Autodesk Inventor part; units mm, degrees
ref_plane "YZ Plane" through (0, 0, 0) normal (1, 0, 0) x (0, 1, 0)
ref_plane "XZ Plane" through (0, 0, 0) normal (0, 1, 0) x (-1, 0, 0)
ref_plane "XY Plane" through (0, 0, 0) normal (0, 0, 1) x (1, 0, 0)
ref_plane "Work Plane1" through (0, 0, 0) normal (0, 0, 1) x (1, 0, 0)
sketch "Sketch1" plane through (0, 0, 0) normal (0, 0, 1) x (1, 0, 0)
  circle A0 centre (0, 0) radius 7.5
  line L0 (-30, 28) -> (-28, 30)
  line L1 (-30, -28) -> (-30, 28)
  line L2 (-28, -30) -> (-30, -28)
  line L3 (28, -30) -> (-28, -30)
  line L4 (30, -28) -> (28, -30)
  line L5 (30, 28) -> (30, -28)
  line L6 (28, 30) -> (30, 28)
  line L7 (-28, 30) -> (28, 30)
  circle A1 centre (-25, 0) radius 1.3
  circle A2 centre (25, 0) radius 1.3
extrude "Extrusion1" add sketch "Sketch1" along normal blind 12 contours A0 | L0 L7 L6 L5 L4 L3 L2 L1 | A1 | A2
sketch "Sketch2" plane through (0, 0, 12) normal (0, 0, 1) x (1, 0, 0)
  point P0 (0, 0)
sketch "Sketch3" plane through (30, -28, 0) normal (1, 0, 0) x (0, 0, -1)
  line L0 (0, 56) -> (0, 0)
  line L1 (0, 56) -> (-12, 56)
  line L2 (-12, 0) -> (-12, 56)
  line L3 (0, 0) -> (-12, 0)
  line L4 (-12, 0) -> (-12, 56)
  line L5 (0, 47.2331) -> (-12, 47.2331)
  line L6 (-12, 47.2331) -> (-12, 36.3051)
  line L7 (-12, 36.3051) -> (0, 36.3051)
  line L8 (0, 36.3051) -> (0, 47.2331)
  line L9 (0, 56) -> (0, 0)
  line L10 (0, 10.2066) -> (-12, 10.2066)
  line L11 (-12, 10.2066) -> (-12, 18.9489)
  line L12 (-12, 18.9489) -> (0, 18.9489)
  line L13 (0, 18.9489) -> (0, 10.2066)
  point P0 (0, 28)
extrude "Extrusion2" add sketch "Sketch3" along normal blind 14 contours L0 L7 L2 L5 | L0 L10 L2 L12
sketch "Sketch4" plane through (30, 19.2331, 12) normal (0, 1, 0) x (1, 0, 0)
  line L0 (0, 0) -> (0, 12)
  line L1 (0, 0) -> (14, 0)
  line L2 (14, 12) -> (14, 0)
  line L3 (0, 12) -> (14, 12)
  circle A0 centre (7, 5) radius 1.5
  point P0 (-30, 12)
  dimension "d4" = 3
extrude "Extrusion3" cut sketch "Sketch4" against normal through all contours A0
pattern_circular "Circular Pattern1" count 2 over 90 about axis through (0, 0, 0) along (0, 0, 1) of "Extrusion2", "Extrusion3"
properties part number "00_XY_stage-CHUO_SEIKI_LD-647-R1-Middle"
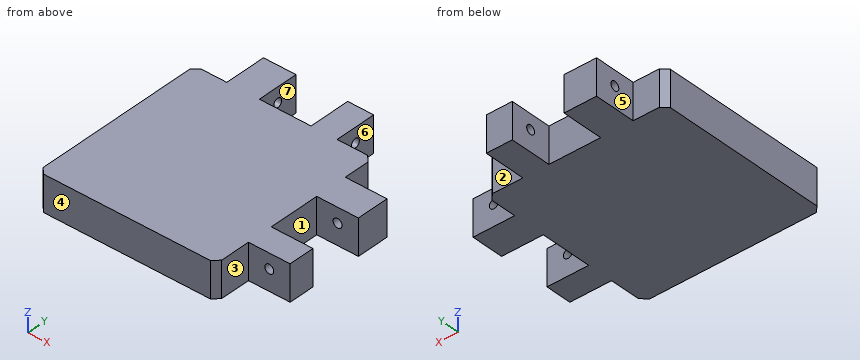
The model under review builds one solid part; all positions refer to its coordinate system, in mm. Face numbers are marked on the shaded views. A direction names the side the tool comes from. Round coordinates to 2 decimals unless told otherwise and drop trailing zeros. Loops run counter-clockwise (first coordinate to the right, second up) from the corner with the lowest first, then second, coordinate; pieces in that order, holes last. Notation, with made-up numbers: (-21, 3) - (-11, 3) arc R33 cw to (-11, 37) - close; hole circle Ø2 at (-29.75, 71.5). An arc over 180 degrees is marked (long way). Write each question's results on one line, items separated by ' | '. Start each with the question number.
Q1. Tool access review of the marked faces 5, 6 and 7: name each direction out of +Z, -Z, +X, -X, +Y, -Y from which nothing blocks a thin tool from reaching the whole face with its end or side.
Q2. Draft analysis for pull direction Y (two halves, no side actions). For the marked faces 1, 2, 3 and 4, state which applies: pulls with the +Y half, pulls with the -Y half, needs draft (parallel to the pull), parting line crosses it, or undercut.
Q3. Take a section at C-C on z = 4. Give the boundary of the cut face in (x, y).
Q4. Take a section at D-D on x = -23.5. Give the boundary of the cut face in (y, z), plus the area to 3 significant figures.
Q5. Take a section at B-B on y = 37. Give the boundary of the cut face in (x, z), plus the area to 3 significant figures.
Q6. Take a section at A-A on x = 34.5. Give the boundary of the cut face in (y, z), plus the area to 3 significant figures.
Q7. Insertion check: P1, Ø2, axis at x = 34, z = 2.5, coming from the -Y side; P2, Ø3, axis at x = 24, z = 7, coming from the +Y side; P3, Ø4.5, axis at y = 24, z = 8.5, coming from the +X side. Each pin has a flat end and moves straight along its axis. Give the tip position at first contact, or say it passes through.
Q8. Wall thickness on line 1 along X through (y, z) = (36.5, 3.75); line 2 along Z through (x, y) = (12, 37); line 3 along Y through (x, z) = (31, 3.75): over which ranges is each line inside the solid? List them lowest first. Write a range as [from, to].
Data:
1) face 5: +Z, -Z, -X, +Y | face 6: +Z, -Z, +X, +Y | face 7: +Z, -Z, +Y
2) face 1: undercut | face 2: pulls with the +Y half | face 3: needs draft | face 4: pulls with the -Y half
3) outline: (-30, -28) - (-28, -30) - (28, -30) - (30, -28) - (30, -17.79) - (44, -17.79) - (44, -9.05) - (30, -9.05) - (30, 8.31) - (44, 8.31) - (44, 19.23) - (30, 19.23) - (30, 28) - (28, 30) - (17.79, 30) - (17.79, 44) - (9.05, 44) - (9.05, 30) - (-8.31, 30) - (-8.31, 44) - (-19.23, 44) - (-19.23, 30) - (-28, 30) - (-30, 28) - close
4) outline: (-30, 0) - (30, 0) - (30, 12) - (-30, 12) - close | area: 720 mm²
5) outline: (-19.23, 0) - (-8.31, 0) - (-8.31, 5.5) - (-19.23, 5.5) - close; (-19.23, 8.5) - (-8.31, 8.5) - (-8.31, 12) - (-19.23, 12) - close; (9.05, 0) - (17.79, 0) - (17.79, 5.5) - (9.05, 5.5) - close; (9.05, 8.5) - (17.79, 8.5) - (17.79, 12) - (9.05, 12) - close | area: 177 mm²
6) outline: (-17.79, 0) - (-9.05, 0) - (-9.05, 12) - (-17.79, 12) - close; (8.31, 0) - (19.23, 0) - (19.23, 12) - (8.31, 12) - close | area: 236 mm²
7) P1: stops at y = -17.79 | P2: stops at y = 30 | P3: stops at x = 30
8) line 1: x = [-19.23, -8.31], [9.05, 17.79] | line 2: z = [0, 5.5], [8.5, 12] | line 3: y = [-17.79, -9.05], [8.31, 19.23]
